Read the model definition and answer for the solid it produces. Units are mm, in the model's axes. A direction names the side the tool comes from. Coordinates: 2 decimals unless noted, no trailing zeros. Write each loop counter-clockwise with the first axis right and the second up, starting at its lowest first coordinate (ties: lowest second). Pieces come first, ordered by that corner, then holes. Notation, with made-up numbers: (-12.75, 40.25) -> (14.25, 40.25) arc R8 cw to (14.25, 45.25) -> close; hole circle Ø11 at (-6, 87.25). An arc over 180 degrees is marked (long way). Answer as a JSON object with one key per item and string values. Group by question number.
(1) Which of the six approach directions +Z, -Z, +X, -X, +Y, -Y give full straight-line access (tool end or side, diameter ignored) to faces 3 (the face through (0, -30, 2)), 4 (the face through (-20.463, 1.43, -1.479)), 5 (the face through (42.952, 26.63, 3.521))?
(2) Find section A-A (y = -53). Give the vertices of the cut face in (x, z), then the cut area to 3 significant figures.
(3) Flat-ended cylindrical pins translate along their axes: P1, Ø3.5, axis at x = 11.5, y = 0, coming from the +Z side; P2, Ø3, axis at x = 24.5, y = 1.5, coming from the -Z side; P3, Ø2.5, axis at x = -22.987, y = 0, coming from the -Z side (3 decimals); P4, Ø13, axis at x = 0, y = 0, coming from the +Z side. Find the tip coordinate at first contact, or state that the pin passes through.
(4) Find section B-B (y = 26.5). Give the vertices of the cut face in (x, z).
(5) Straight lines are drawn through the part: L1, parallel to Y at x = 0, z = 3.05; L2, parallel to Y at x = -20.5, z = -2.5; L3, parallel to Y at x = 8, z = 4.5. For each, find the intervals that lie inside material, in ascending order.
(6) For a pull along Y with two mould halves and no side action, classify faces 1 (the face through (26.76, -51.46, 2.46)), 2 (the face through (11, -3.5, 3)) as +Y half, -Y half, draft (parallel to the pull), parting line (faces both ways), or undercut.
(7) Find section C-C (x = 0). Count the separate pieces of the cut face and the enclosed holes in it, then the cut area to 3 significant figures.
from build123d import *

# Parameters (mm, degrees)
SKETCH1_R                = 58
SKETCH1_R_2              = 8.2
SKETCH1_R_3              = 1.7
BOSS_EXTRUDE1_DEPTH      = 5
SKETCH4_W                = 30.6
SKETCH4_H                = 7
CUT_EXTRUDE2_DEPTH       = 4
CUT_EXTRUDE3_DEPTH       = 4
SKETCH6_R                = 1.7
CUT_EXTRUDE4_DEPTH       = 83.758685345
SKETCH7_R                = 2.95
CUT_EXTRUDE5_DEPTH       = 3
SKETCH8_R                = 1.7
CUT_EXTRUDE6_DEPTH       = 83.758685345
BOSS_EXTRUDE2_DEPTH      = 3
BOSS_EXTRUDE2_DEPTH_BACK = 10
CUT_EXTRUDE7_DEPTH       = 84.210576251
CUT_EXTRUDE7_DEPTH_BACK  = 84.210576251
FILLET1_R                = 1
SKETCH11_R               = 7
BOSS_EXTRUDE3_DEPTH      = 3


with BuildPart() as part:
    # Sketch1 → Boss-Extrude1 (new body)
    with BuildSketch(Plane.XY):
        Circle(SKETCH1_R)
        Circle(SKETCH1_R_2, mode=Mode.SUBTRACT)
        with Locations((0, -53)):
            Circle(SKETCH1_R_3, mode=Mode.SUBTRACT)
        with Locations((-45.899346401, 26.5)):
            Circle(SKETCH1_R_3, mode=Mode.SUBTRACT)
        with Locations((45.899346401, 26.5)):
            Circle(SKETCH1_R_3, mode=Mode.SUBTRACT)
    extrude(amount=BOSS_EXTRUDE1_DEPTH)

    # Sketch3 → Revolve1 (revolve)
    with BuildSketch(Plane(origin=(0, 0, 0), x_dir=(1, 0, 0), z_dir=(0, 1, 0)), mode=Mode.PRIVATE) as revolve1_sk:
        Polygon((-8.2, 0), (-18, 0), (-12, 6), (-5, 6), (-5, 4), (-8.2, 4), align=None)
    revolve(revolve1_sk.sketch.rotate(Axis((0, 0, 0), (0, 0, -1)), 180), axis=Axis((0, 0, 0), (0, 0, -1)))

    # Sketch4 → Cut-Extrude2 (cut)
    with BuildSketch(Plane.XY.offset(5)):
        Rectangle(SKETCH4_W, SKETCH4_H)
    extrude(amount=-CUT_EXTRUDE2_DEPTH, mode=Mode.SUBTRACT)

    # Sketch5 → Cut-Extrude3 (cut)
    with BuildSketch(Plane(origin=(0, 0, -6), x_dir=(-1, 0, 0), z_dir=(0, 0, -1))):
        Polygon((-11, 3.35), (-13.901185103, 1.675), (-13.901185103, -1.675), (-11, -3.35), (-8.098814897, -1.675), (-8.098814897, 1.675), align=None)
        Polygon((8.098814897, -1.675), (8.098814897, 1.675), (11, 3.35), (13.901185103, 1.675), (13.901185103, -1.675), (11, -3.35), align=None)
    extrude(amount=-CUT_EXTRUDE3_DEPTH, mode=Mode.SUBTRACT)

    # Sketch6 → Cut-Extrude4 (cut, through all)
    with BuildSketch(Plane(origin=(0, 0, -6), x_dir=(-1, 0, 0), z_dir=(0, 0, -1))):
        with Locations((-11, 0)):
            Circle(SKETCH6_R)
        with Locations(Location((11, 0, 0), (0, 0, 180))):
            Circle(SKETCH6_R)
    extrude(amount=-CUT_EXTRUDE4_DEPTH, mode=Mode.SUBTRACT)

    # Sketch7 → Cut-Extrude5 (cut)
    with BuildSketch(Plane.XY.offset(5)):
        with Locations((-45.899346401, 26.5)):
            Circle(SKETCH7_R)
        with Locations((45.899346401, 26.5)):
            Circle(SKETCH7_R)
        with Locations((0, -53)):
            Circle(SKETCH7_R)
    extrude(amount=-CUT_EXTRUDE5_DEPTH, mode=Mode.SUBTRACT)

    # Sketch8 → Cut-Extrude6 (cut, through all)
    with BuildSketch(Plane.XY.offset(5)):
        with Locations((22.987, 0)):
            Circle(SKETCH8_R)
        with Locations((-22.987, 0)):
            Circle(SKETCH8_R)
    extrude(amount=-CUT_EXTRUDE6_DEPTH, mode=Mode.SUBTRACT)

    # Sketch9 → Boss-Extrude2 (add, two sides: drawn at the far end of the back side and taken through both)
    with BuildSketch(Plane(origin=(0, 0, -6), x_dir=(-1, 0, 0), z_dir=(0, 0, -1)).offset(-BOSS_EXTRUDE2_DEPTH_BACK)):
        with BuildLine():
            ThreePointArc((33, 0), (22.294476851, 24.330152115), (-2.876139511, 32.874425037))
            Line((-2.876139511, 32.874425037), (-2.788983768, 31.878230339))
            ThreePointArc((-2.788983768, 31.878230339), (21.618886644, 23.592874778), (32, 0))
            ThreePointArc((32, 0), (31.969543091, -1.395820396), (31.878230339, -2.788983768))
            Line((31.878230339, -2.788983768), (32.874425037, -2.876139511))
            ThreePointArc((32.874425037, -2.876139511), (32.968591312, -1.439439783), (33, 0))
        make_face()
    extrude(amount=BOSS_EXTRUDE2_DEPTH + BOSS_EXTRUDE2_DEPTH_BACK)

    # Sketch10 → Cut-Extrude7 (cut, two sides: drawn at the far end of the back side and taken through both)
    with BuildSketch(Plane.XY.offset(5).offset(-CUT_EXTRUDE7_DEPTH_BACK)):
        with BuildLine():
            ThreePointArc((18.471052989, -23.639378196), (-0.261796154, -29.998857691), (-18.880803933, -23.313413367))
            ThreePointArc((-18.880803933, -23.313413367), (-23.803462517, -23.830551311), (-23.286324737, -28.753209912))
            ThreePointArc((-23.286324737, -28.753209912), (-0.322881815, -36.998591153), (22.780965409, -29.155233064))
            ThreePointArc((22.780965409, -29.155233064), (23.383936613, -24.242349436), (18.471052989, -23.639378196))
        make_face()
    extrude(amount=CUT_EXTRUDE7_DEPTH + CUT_EXTRUDE7_DEPTH_BACK, mode=Mode.SUBTRACT)

    # Fillet1
    fillet1_edges = [part.edges().sort_by_distance(p)[0] for p in [
        (-0.261796154, -29.998857691, 0),
        (23.383936613, -24.242349436, 0),
        (-0.322881815, -36.998591153, 0),
        (-23.803462517, -23.830551311, 0),
        (-23.803462517, -23.830551311, 5),
        (-0.322881815, -36.998591153, 5),
        (23.383936613, -24.242349436, 5),
        (-0.261796154, -29.998857691, 5),
    ]]
    fillet(fillet1_edges, radius=FILLET1_R)

    # Sketch11 → Boss-Extrude3 (add)
    # profile 1 of 2: a face of its own
    with BuildSketch(Plane(origin=(0, 0, 0), x_dir=(-1, 0, 0), z_dir=(0, 0, -1))):
        with Locations(Location((-22.987, 0, 0), (0, 0, 321.943969813))):
            Circle(SKETCH11_R)
        Polygon((-24.662, 2.901185103), (-26.337, 0), (-24.662, -2.901185103), (-21.312, -2.901185103), (-19.637, 0), (-21.312, 2.901185103), align=None, mode=Mode.SUBTRACT)
    # profile 2 of 2: a face of its own
    with BuildSketch(Plane(origin=(0, 0, 0), x_dir=(-1, 0, 0), z_dir=(0, 0, -1))):
        with Locations(Location((22.987, 0, 0), (0, 0, 180))):
            Circle(SKETCH11_R)
        Polygon((19.637, 0), (21.312, 2.901185103), (24.662, 2.901185103), (26.337, 0), (24.662, -2.901185103), (21.312, -2.901185103), align=None, mode=Mode.SUBTRACT)
    extrude(amount=BOSS_EXTRUDE3_DEPTH)


solid = part.part
Results below:
{
 "1": {"face 3": "+Z, -Z", "face 4": "-Z", "face 5": "+Z"},
 "2": {"outline": "(-23.56, 0) -> (-1.7, 0) -> (-1.7, 2) -> (-2.95, 2) -> (-2.95, 5) -> (-23.56, 5) -> close; (1.7, 0) -> (23.56, 0) -> (23.56, 5) -> (2.95, 5) -> (2.95, 2) -> (1.7, 2) -> close", "area": "211 mm2"},
 "3": {"P1": "stops at z = 1", "P2": "stops at z = -3", "P3": "passes through", "P4": "stops at z = -4"},
 "4": {"outline": "(-51.59, 0) -> (-47.6, 0) -> (-47.6, 2) -> (-48.85, 2) -> (-48.85, 5) -> (-51.59, 5) -> close; (-44.2, 0) -> (-19.67, 0) -> (-19.67, -9) -> (-17.94, -9) -> (-17.94, 0) -> (44.2, 0) -> (44.2, 2) -> (42.95, 2) -> (42.95, 5) -> (-42.95, 5) -> (-42.95, 2) -> (-44.2, 2) -> close; (47.6, 0) -> (51.59, 0) -> (51.59, 5) -> (48.85, 5) -> (48.85, 2) -> (47.6, 2) -> close"},
 "5": {"L1": "y = -58 to -55.95, -50.05 to -37, -30 to -8.2, 8.2 to 58", "L2": "y = -6.54 to -1.49, 1.49 to 6.54, 24.57 to 25.86", "L3": "y = -57.45 to -36.26, -28.77 to -3.5, 3.5 to 57.45"},
 "6": {"face 1": "parting line", "face 2": "undercut"},
 "7": {"separate pieces": "4", "enclosed holes": "0", "area": "541 mm2"}
}
